The figure shows three views and two pictorial views of one solid part (mm, origin at its lowest corner). Answer the questions. A direction names the side the tool comes from. Coordinates: 2 decimals unless noted, no trailing zeros. Write each loop counter-clockwise with the first axis right and the second up, starting at its lowest first coordinate (ties: lowest second). Pieces come first, ordered by that corner, then holes.
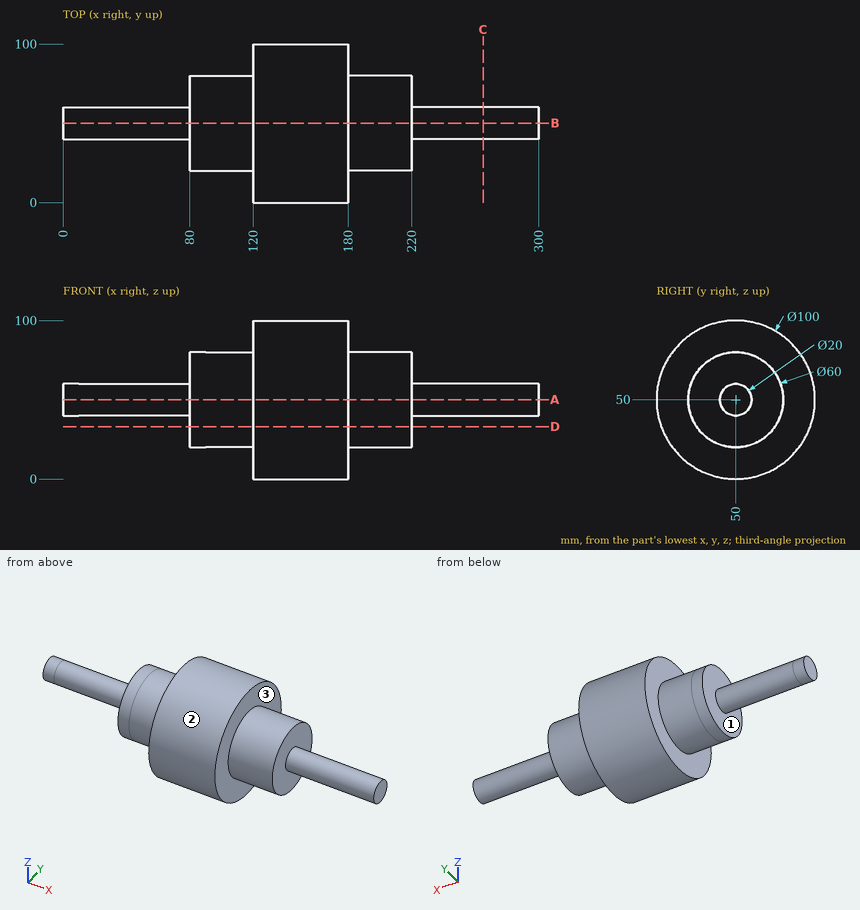
Q1. Which of the six approach directions +Z, -Z, +X, -X, +Y, -Y give full straight-line access (tool end or side, diameter ignored) to the marked faces 1, 2 and 3?
Answers below:
face 1: -X
face 2: +X, -X
face 3: +X
Q2. Given pin 1 (6 mm diameter, centred on y = 68, z = 43, fed in from -X); pin 2 (1.5 mm diameter, centred on y = 74.5, z = 68.5, fed in from +X); pin 3 (6 mm diameter, centred on x = 259, z = 44, fed in from -Y), each flat-ended and moving along its own axis, determine where each tip first touches the part or whether it passes through.
Answers below:
pin 1: stops at x = 80
pin 2: stops at x = 220
pin 3: stops at y = 40.46
Q3. The part is cut by section A-A, the plane z = 50. Write down the section's boundary in (x, y).
Answers below:
outline: (0, 40) - (80, 40) - (80, 20) - (120, 20) - (120, 0) - (180, 0) - (180, 20) - (220, 20) - (220, 40) - (300, 40) - (300, 60) - (220, 60) - (220, 80) - (180, 80) - (180, 100) - (120, 100) - (120, 80) - (80, 80) - (80, 60) - (0, 60) - close
Q4. The part is cut by section C-C, the plane x = 265. Write down the section's boundary in (y, z), then the cut area to 3 significant figures.
Answers below:
outline: circle Ø20 at (50, 50)
area: 314 mm2
Q5. Find the intervals of material crossed by probe 1 along X at (y, z) = (72.5, 40); probe 2 along Y at (x, z) = (135, 90); probe 3 along X at (y, z) = (60, 13), in increasing order.
Answers below:
probe 1: x = 80 to 220
probe 2: y = 20 to 80
probe 3: x = 120 to 180
Q6. The part is cut by section D-D, the plane z = 33. Write down the section's boundary in (x, y), then the cut area to 3 significant figures.
Answers below:
outline: (80, 25.28) - (120, 25.28) - (120, 2.98) - (180, 2.98) - (180, 25.28) - (220, 25.28) - (220, 74.72) - (180, 74.72) - (180, 97.02) - (120, 97.02) - (120, 74.72) - (80, 74.72) - close
area: 9,600 mm2
